Here's the drawing with two shaded views (mm, measured from the low corner). I have some questions. A direction names the side the tool comes from. Give positions to 0.01 mm unless a question says otherwise; leave off trailing zeros. Order: outer loops, then holes, each group sorted by start corner. A loop starts at its lowest first (then second) coordinate and runs counter-clockwise, first axis right, second up. Notation, with made-up numbers: (-35.75, 49) - (-27.75, 49) arc R28 cw to (-27.75, 76) - close; hole circle Ø7 at (-20.75, -36.75). An arc over 180 degrees is marked (long way). Use one line per item in the form item = value. Start each with the question number.
1) We'd pull the mould along X, two halves only. Please class the marked faces 1, 2 and 3: released by +X, released by -X, zero draft, split by the parting line, or undercut.
2) For pin 1 (7 mm diameter, centred on x = 127, y = 4, fed in from +Z) (1 decimal), with a flat end and sliding along its axis, tell me the tip position at first contact or that it passes through.
3) Suppose I cut it at A-A, the plane y = 26. Write out the boundary of the cut face in (x, z), and give its area (3 significant figures).
4) Suppose I cut it at D-D, the plane z = 71. Write out the boundary of the cut face in (x, y).
5) Please list where these lines run through material, in increasing order: probe 1 along X at (y, z) = (40, 71); probe 2 along Y at (x, z) = (14, 50.5).
6) Which directions (+Z, -Z, +X, -X, +Y, -Y) give clear straight access to the entire face, cutting with the end or side of a thin tool? Please do the marked faces 4 and 5.
7) Suppose I cut it at B-B, the plane z = 25. Write out the boundary of the cut face in (x, y), and give its area (3 significant figures).
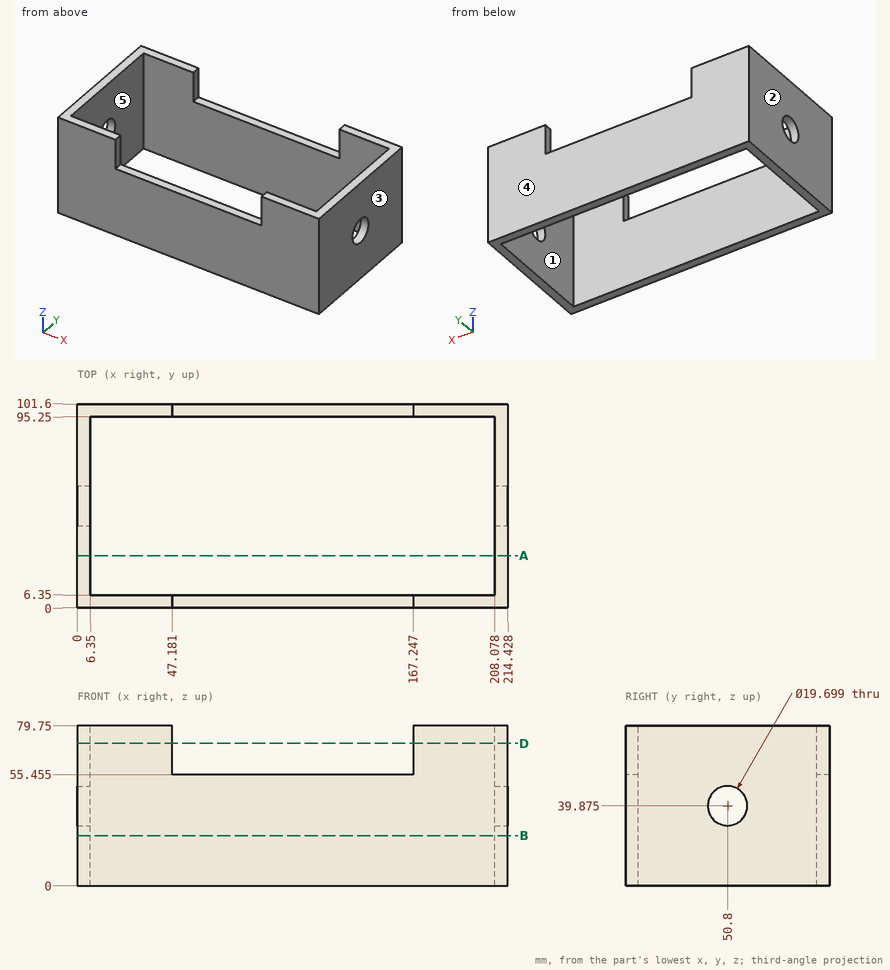
Result sheet:
q1.face_1 = undercut
q1.face_2 = released by -X
q1.face_3 = released by +X
q2.pin_1 = 55.5
q3.outline = (0, 0) - (6.35, 0) - (6.35, 79.75) - (0, 79.75) - close; (208.08, 0) - (214.43, 0) - (214.43, 79.75) - (208.08, 79.75) - close
q3.area = 1,010 mm²
q4.outline = (0, 0) - (47.18, 0) - (47.18, 6.35) - (6.35, 6.35) - (6.35, 95.25) - (47.18, 95.25) - (47.18, 101.6) - (0, 101.6) - close; (167.25, 0) - (214.43, 0) - (214.43, 101.6) - (167.25, 101.6) - (167.25, 95.25) - (208.08, 95.25) - (208.08, 6.35) - (167.25, 6.35) - close
q5.probe_1 = 0 to 6.35, 208.08 to 214.43
q5.probe_2 = 0 to 6.35, 95.25 to 101.6
q6.face_4 = +Z, -Z, +X, -X, +Y
q6.face_5 = +Z, -Z
q7.outline = (0, 0) - (214.43, 0) - (214.43, 101.6) - (0, 101.6) - close; hole (6.35, 6.35) - (208.08, 6.35) - (208.08, 95.25) - (6.35, 95.25) - close
q7.area = 3,850 mm²
